```python
from build123d import *

# Parameters (mm, degrees)
SKETCH1_R           = 3
SKETCH1_W           = 40.5
SKETCH1_H           = 20.5
BOSS_EXTRUDE1_DEPTH = 5
FILLET2_R           = 20
BOSS_EXTRUDE2_START = -5
SKETCH3_R           = 19.722379498
SKETCH3_R_2         = 3
BOSS_EXTRUDE2_DEPTH = 5
FILLET3_R           = 10
SKETCH4_R           = 1
CUT_EXTRUDE1_DEPTH  = 6
SKETCH5_R           = 1.5
CUT_EXTRUDE2_DEPTH  = 6
SKETCH6_R           = 4.5
CUT_EXTRUDE3_DEPTH  = 6
CIRPATTERN1_COUNT   = 6


with BuildPart() as part:
    # Sketch1 → Boss-Extrude1 (new body)
    with BuildSketch(Plane.XY):
        Polygon((75, 20), (75, -20), (-75, -15), (-78, -15), (-78, 15), (-75, 15), align=None)
        with Locations((67, 0)):
            Circle(SKETCH1_R, mode=Mode.SUBTRACT)
        with Locations((-50, 0)):
            Rectangle(SKETCH1_W, SKETCH1_H, mode=Mode.SUBTRACT)
    extrude(amount=BOSS_EXTRUDE1_DEPTH)

    # Fillet2
    # the kernel refuses this fillet: 20 mm, written as the material it takes off along each edge
    with BuildSketch(Plane(origin=(75, -20, -51.694436733), x_dir=(0, 1, 0), z_dir=(0, 0, 1))) as fillet2_piece_1:
        with BuildLine():
            CenterArc((FILLET2_R * 1.03388873465, FILLET2_R), FILLET2_R, 178.090847567, 91.909152433)
            Line((FILLET2_R * 0.0344438276744, FILLET2_R * 1.03331483023), (0, 0))
            Line((0, 0), (FILLET2_R * 1.03388873465, 0))
        make_face()
    extrude(amount=108.388873465, mode=Mode.SUBTRACT)
    with BuildSketch(Plane(origin=(75, 20, -51.694436733), x_dir=(0, -1, 0), z_dir=(0, 0, 1))) as fillet2_piece_2:
        with BuildLine():
            CenterArc((FILLET2_R * 1.03388873465, -FILLET2_R), FILLET2_R, 90, 91.909152433)
            Line((FILLET2_R * 0.0344438276744, -FILLET2_R * 1.03331483023), (0, 0))
            Line((0, 0), (FILLET2_R * 1.03388873465, 0))
        make_face()
    extrude(amount=108.388873465, mode=Mode.SUBTRACT)

    # Sketch3 → Boss-Extrude2 (add)
    with BuildSketch(Plane.XY.offset(5).offset(BOSS_EXTRUDE2_START)):
        with Locations((67, 0)):
            Circle(SKETCH3_R)
        with Locations((67, 0)):
            Circle(SKETCH3_R_2, mode=Mode.SUBTRACT)
    extrude(amount=BOSS_EXTRUDE2_DEPTH)

    # Fillet3
    fillet3_edges = [part.edges().sort_by_distance(p)[0] for p in [
        (-78, 15, 2.5),
        (-78, -15, 2.5),
        (60.390814278, -18.582005197, 2.5),
        (60.390814278, 18.582005197, 2.5),
    ]]
    fillet(fillet3_edges, radius=FILLET3_R)

    # Sketch4 → Cut-Extrude1 (cut)
    with BuildSketch(Plane(origin=(0, 0, 0), x_dir=(-1, 0, 0), z_dir=(0, 0, -1))):
        with Locations((25.6, -5)):
            Circle(SKETCH4_R)
        with Locations(Location((25.6, 5, 0), (0, 0, 180))):
            Circle(SKETCH4_R)
        with Locations((74.4, 5)):
            Circle(SKETCH4_R)
        with Locations(Location((74.4, -5, 0), (0, 0, 180))):
            Circle(SKETCH4_R)
    extrude(amount=-CUT_EXTRUDE1_DEPTH, mode=Mode.SUBTRACT)

    # Sketch5 → Cut-Extrude2 (cut)
    with BuildSketch(Plane.XY.offset(5)):
        with Locations((67, 13.5)):
            Circle(SKETCH5_R)
    cut_extrude2 = extrude(amount=-CUT_EXTRUDE2_DEPTH, mode=Mode.SUBTRACT)

    # Sketch6 → Cut-Extrude3 (cut)
    with BuildSketch(Plane.XY.offset(5)):
        with Locations((67, 0)):
            Circle(SKETCH6_R)
    extrude(amount=-CUT_EXTRUDE3_DEPTH, mode=Mode.SUBTRACT)

    # CirPattern1: Cut-Extrude2 ×6 about axis
    cirpattern1_axis = Axis((67, 0, 0), (0, 0, 1))
    for i in range(1, CIRPATTERN1_COUNT):
        add(cut_extrude2.rotate(cirpattern1_axis, i * 360 / CIRPATTERN1_COUNT), mode=Mode.SUBTRACT)


solid = part.part
```
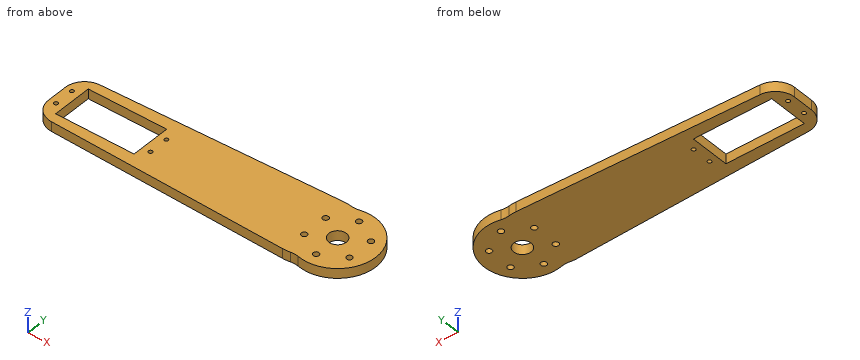
Check sheet for the modelled part. Datum: model origin and axes. Units: mm. Give positions to 0.01 mm unless a question says otherwise; leave off trailing zeros. Write each loop counter-clockwise with the first axis right and the second up, starting at its lowest first coordinate (ties: lowest second). Pieces come first, ordered by that corner, then holes.
Item 1: Cross-section at C-C (z = 2.6). Count the separate pieces of the cut face and the enclosed holes in it, and give its area (3 significant figures).
Item 2: Cross-section at A-A (x = 67). Enter the section's corners in (y, z), and give its area (3 significant figures).
Item 3: Cross-section at B-B (x = 39). Enter the section's corners in (y, z).
Item 4: Gauge pin test, flat ends, axial feed: pin 1 (3 mm diameter, centred on x = 39.5, z = 1.5, fed in from -Y); pin 2 (1.5 mm diameter, centred on x = -56, z = 3.5, fed in from -Y); pin 3 (1.5 mm diameter, centred on x = -48, z = 3, fed in from +Y) (3 decimals). Record the tip position at first contact, or that the pin passes through.
Item 5: Scan lines: L1, parallel to X at y = -0.5, z = 0.6; L2, parallel to Y at x = 67, z = 2.8; L3, parallel to Y at x = -74.4, z = 2.3. Record each from-to range of solid material in increasing order.
Report:
1. separate pieces: 1
1. enclosed holes: 12
1. area: 4,640 mm2
2. outline: (-19.72, 0) - (-15, 0) - (-15, 5) - (-19.72, 5) - close; (-12, 0) - (-4.5, 0) - (-4.5, 5) - (-12, 5) - close; (4.5, 0) - (12, 0) - (12, 5) - (4.5, 5) - close; (15, 0) - (19.72, 0) - (19.72, 5) - (15, 5) - close
2. area: 122 mm2
3. outline: (-18.8, 0) - (18.8, 0) - (18.8, 5) - (-18.8, 5) - close
4. pin 1: stops at y = -18.87
4. pin 2: stops at y = -15.66
4. pin 3: stops at y = 15.925
5. L1: x = -78 to -70.25, -29.75 to 62.53, 71.47 to 86.72
5. L2: y = -19.72 to -15, -12 to -4.5, 4.5 to 12, 15 to 19.72
5. L3: y = -12.91 to -6, -4 to 4, 6 to 12.91
